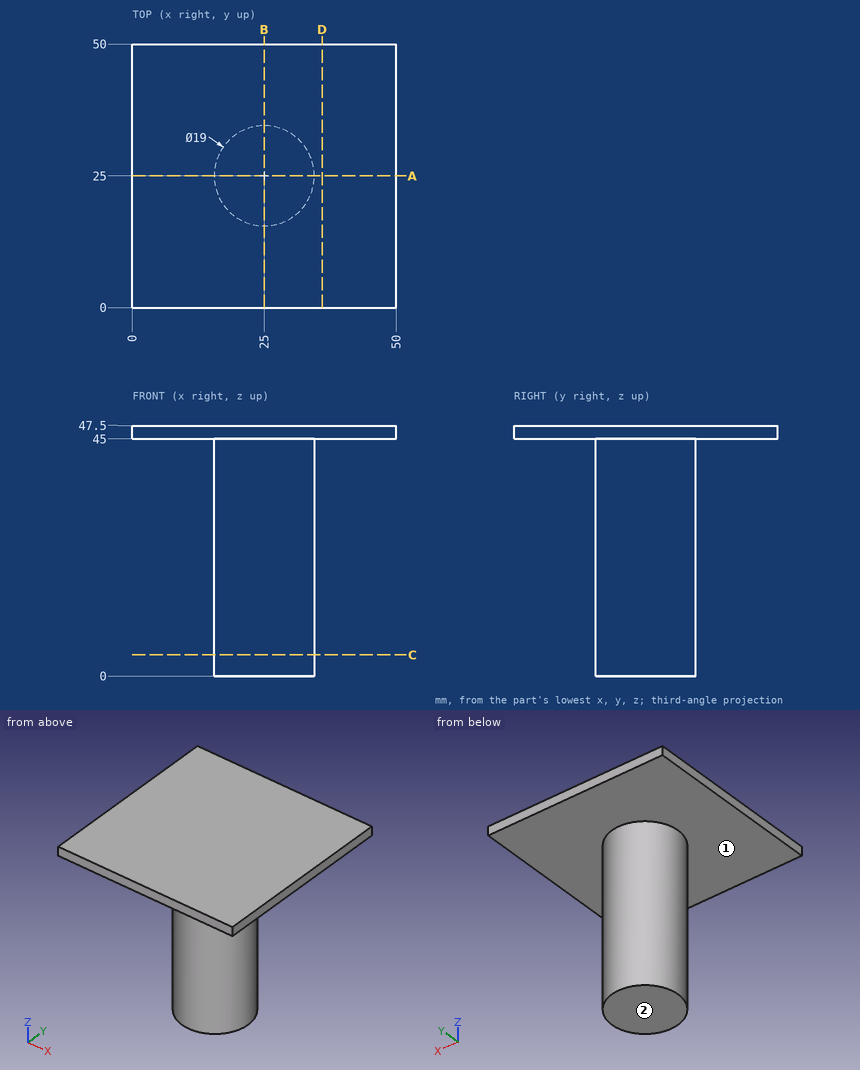
Here's the drawing with two shaded views (mm, measured from the low corner). I have some questions. A direction names the side the tool comes from. Coordinates: 2 decimals unless noted, no trailing zeros. Write each loop counter-clockwise with the first axis right and the second up, starting at its lowest first coordinate (ties: lowest second). Pieces come first, ordered by that corner, then holes. Notation, with made-up numbers: (41.5, 22.5) -> (97.5, 22.5) arc R22 cw to (97.5, 31.5) -> close; hole circle Ø9 at (-23, 52.5). An arc over 180 degrees is marked (long way). Write item = value, one per line. Start each with the question number.
(1) I want a section at C-C (z = 4). Please give me the cut outline in (x, y), plus the area to 3 significant figures.
(2) I want a section at D-D (x = 36). Please give me the cut outline in (y, z).
(3) Will this pin go through, and if not, where does the flat tip stop? pin 1 (4 mm diameter, centred on y = 16.5, z = 12.5, fed in from +X).
(4) I want a section at A-A (y = 25). Please give me the cut outline in (x, z).
(5) I need wall thicknesses on line 1 (Z direction, x = 30.5, y = 3); line 2 (Y direction, x = 25, z = 10); line 3 (X direction, y = 25.5, z = 38.5). Which ranges of each line are inside material? Lowest first, please. Write a range as [from, to].
(6) Which directions (+Z, -Z, +X, -X, +Y, -Y) give clear straight access to the entire face, cutting with the end or side of a thin tool? Please do the marked faces 1 and 2.
Result set:
q1.outline = circle Ø19 at (25, 25)
q1.area = 284 mm2
q2.outline = (0, 45) -> (50, 45) -> (50, 47.5) -> (0, 47.5) -> close
q3.pin_1 = 31.93
q4.outline = (0, 45) -> (15.5, 45) -> (15.5, 0) -> (34.5, 0) -> (34.5, 45) -> (50, 45) -> (50, 47.5) -> (0, 47.5) -> close
q5.line_1 = [45, 47.5]
q5.line_2 = [15.5, 34.5]
q5.line_3 = [15.51, 34.49]
q6.face_1 = -Z
q6.face_2 = -Z, +X, -X, +Y, -Y
